Read the model definition and answer for the solid it produces. Units are mm, in the model's axes. A direction names the side the tool comes from. Coordinates: 2 decimals unless noted, no trailing zeros. Loops run counter-clockwise (first coordinate to the right, second up) from the corner with the lowest first, then second, coordinate; pieces in that order, holes last.
Q1. Which of the six approach directions +Z, -Z, +X, -X, +Y, -Y give full straight-line access (tool end or side, diameter ignored) to faces 1 (the face through (0, 37, -22.5)), 2 (the face through (-22.5, 37, 0)), 3 (the face through (22.5, 37, 0)), 4 (the face through (-24, -3, 0)), 5 (the face through (0, 78, 20.5))?
Q2. Section A-A (x = 12.5) is taken. Give the vertices of the cut face in (y, z), then the cut area to 3 significant figures.
Q3. Flat-ended cylindrical pins translate along their axes: P1, Ø10, axis at x = 0, y = 16.5, coming from the +Z side; P2, Ø2.5, axis at y = 79, z = -9, coming from the -X side; P3, Ø2, axis at x = 11.5, y = 29, coming from the -Z side. Find the tip coordinate at first contact, or state that the pin passes through.
Q4. Straight lines are drawn through the part: line 1 (Z direction, x = 1, y = 41); line 2 (X direction, y = 76.5, z = -18.5). For each, find the intervals that lie inside material, in ascending order.
Q5. Section C-C (y = 47.5) is taken. Give the vertices of the cut face in (x, z).
Q6. Section B-B (z = 4) is taken. Give the vertices of the cut face in (x, y).
from build123d import *

# Parameters (mm, degrees)
F0_W     = 48
F0_H     = 48
F1_DEPTH = 6
F2_W     = 45
F2_H     = 45
F3_DEPTH = 74.5
F4_W     = 41
F4_H     = 41
F5_DEPTH = 8


with BuildPart() as f1:
    # F0 (on Front) → F1 (new body)
    with BuildSketch(Plane.XZ):
        Rectangle(F0_W, F0_H)
    extrude(amount=F1_DEPTH)

    # F2 (on face) → F3 (join)
    with BuildSketch(Plane(origin=(0, 0, 0), x_dir=(-1, 0, 0), z_dir=(0, 1, 0))):
        Rectangle(F2_W, F2_H)
    extrude(amount=F3_DEPTH)

    # F4 (on face) → F5 (join)
    with BuildSketch(Plane(origin=(0, 74.5, 0), x_dir=(-1, 0, 0), z_dir=(0, 1, 0))):
        Rectangle(F4_W, F4_H)
    extrude(amount=F5_DEPTH)


solid = f1.part
Numbers:
1. face 1: -Z, +X, -X, +Y
1. face 2: +Z, -Z, -X, +Y
1. face 3: +Z, -Z, +X, +Y
1. face 4: +Z, -Z, -X, +Y, -Y
1. face 5: +Z, +X, -X, +Y
2. outline: (-6, -24) - (0, -24) - (0, -22.5) - (74.5, -22.5) - (74.5, -20.5) - (82.5, -20.5) - (82.5, 20.5) - (74.5, 20.5) - (74.5, 22.5) - (0, 22.5) - (0, 24) - (-6, 24) - close
2. area: 3,970 mm2
3. P1: stops at z = 22.5
3. P2: stops at x = -20.5
3. P3: stops at z = -22.5
4. line 1: z = -22.5 to 22.5
4. line 2: x = -20.5 to 20.5
5. outline: (-22.5, -22.5) - (22.5, -22.5) - (22.5, 22.5) - (-22.5, 22.5) - close
6. outline: (-24, -6) - (24, -6) - (24, 0) - (22.5, 0) - (22.5, 74.5) - (20.5, 74.5) - (20.5, 82.5) - (-20.5, 82.5) - (-20.5, 74.5) - (-22.5, 74.5) - (-22.5, 0) - (-24, 0) - close
